CAD build for the part. Positions are in the model's coordinates, mm. Face numbers are marked on the shaded views. A direction names the side the tool comes from. Give positions to 0.01 mm unless a question says otherwise; leave off trailing zeros. Loops run counter-clockwise (first coordinate to the right, second up) from the corner with the lowest first, then second, coordinate; pieces in that order, holes last.
Item 1: Saw through at B-B on y = 1.5. Give the cut face in (x, z), plus the area to 3 significant figures.
Item 2: Probe probe 1 along X at (y, z) = (0.7, -29); probe 2 along X at (y, z) = (1.5, -29.5); probe 3 along Y at (x, z) = (37.5, -16.85). List the from-to ranges inside material, lowest first.
Item 3: Which spindle directions (+Z, -Z, +X, -X, +Y, -Y) get a long thin tool onto all of the face, cutting with end or side? Do the marked faces 1, 2 and 3. Say none if no direction does.
Item 4: Drop flat-ended pins along their axis: P1, Ø13, axis at y = 9, z = -20, coming from the +X side; P2, Ø4.5, axis at x = 20.5, y = 17, coming from the -Z side; P3, Ø2.5, axis at x = 49, z = -6, coming from the +Y side; P4, Ø5, axis at x = 17.5, y = 14.5, coming from the +Z side. Give the stop position or say it passes through.
Item 5: Saw through at D-D on x = 17.5. Give the cut face in (y, z), plus the area to 3 significant figures.
Item 6: Saw through at A-A on x = 6. Give the cut face in (y, z), plus the area to 3 significant figures.
Item 7: Saw through at C-C on z = -29. Give the cut face in (x, y).
from build123d import *

# Parameters (mm, degrees)
SKETCH_1_W          = 55
SKETCH_1_H          = 35
EXTRUDE_1_DEPTH     = 3
SKETCH_2_R          = 1.6
CUT_EXTRUDE_1_DEPTH = 3
FILLET_1_R          = 3
SKETCH_3_W          = 30
SKETCH_3_H          = 4
EXTRUDE_2_DEPTH     = 19
CHAMFER_1_SIZE      = 4
SKETCH_4_R          = 1.6
CUT_EXTRUDE_2_DEPTH = 19
FILLET_3_R          = 4


with BuildPart() as part:
    # 草图1 → 凸台-拉伸1 (new body)
    with BuildSketch(Plane(origin=(0, 0, 0), x_dir=(1, 0, 0), z_dir=(0, 1, 0))):
        with Locations((27.5, 17.5)):
            Rectangle(SKETCH_1_W, SKETCH_1_H)
    extrude(amount=EXTRUDE_1_DEPTH)

    # 草图2 → 切除-拉伸1 (cut)
    with BuildSketch(Plane(origin=(0, 3, 0), x_dir=(1, 0, 0), z_dir=(0, 1, 0))):
        with Locations(Location((6, 29, 0), (0, 0, 270))):
            Circle(SKETCH_2_R)
        with Locations(Location((49, 29, 0), (0, 0, 270))):
            Circle(SKETCH_2_R)
        with Locations(Location((49, 6, 0), (0, 0, 270))):
            Circle(SKETCH_2_R)
        with Locations(Location((6, 6, 0), (0, 0, 270))):
            Circle(SKETCH_2_R)
    extrude(amount=-CUT_EXTRUDE_1_DEPTH, mode=Mode.SUBTRACT)

    # 圆角1
    fillet_1_edges = [part.edges().sort_by_distance(p)[0] for p in [
        (0, 1.5, -35),
        (55, 1.5, -35),
        (55, 1.5, 0),
        (0, 1.5, 0),
    ]]
    fillet(fillet_1_edges, radius=FILLET_1_R)

    # 草图3 → 凸台-拉伸2 (add)
    with BuildSketch(Plane(origin=(0, 3, 0), x_dir=(1, 0, 0), z_dir=(0, 1, 0))):
        with Locations((27.5, 17.5)):
            Rectangle(SKETCH_3_W, SKETCH_3_H)
    extrude(amount=EXTRUDE_2_DEPTH)

    # 倒角1
    chamfer_1_edges = [part.edges().sort_by_distance(p)[0] for p in [
        (27.5, 3, -15.5),
        (27.5, 3, -19.5),
    ]]
    chamfer(chamfer_1_edges, length=CHAMFER_1_SIZE)

    # 草图4 → 切除-拉伸2 (cut)
    with BuildSketch(Plane(origin=(0, 0, -19.5), x_dir=(-1, 0, 0), z_dir=(0, 0, -1))):
        with Locations((-37.5, 14.5)):
            Circle(SKETCH_4_R)
        with Locations((-17.5, 14.5)):
            Circle(SKETCH_4_R)
    extrude(amount=-CUT_EXTRUDE_2_DEPTH, mode=Mode.SUBTRACT)

    # 圆角3
    fillet_3_edges = [part.edges().sort_by_distance(p)[0] for p in [
        (12.5, 22, -17.5),
        (42.5, 22, -17.5),
    ]]
    fillet(fillet_3_edges, radius=FILLET_3_R)


solid = part.part
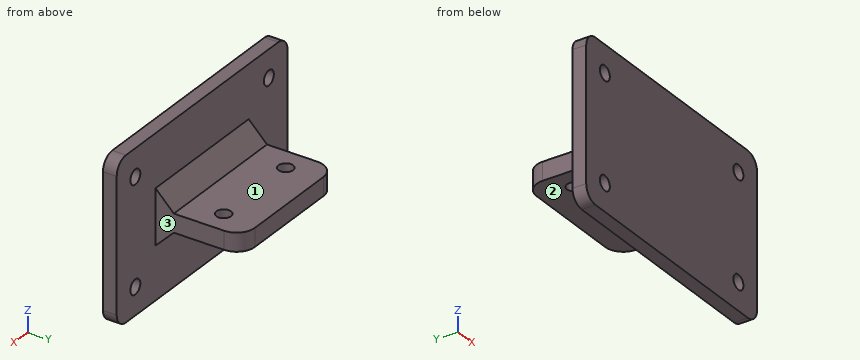
Results below:
1. outline: (0, -32) arc R3 ccw to (3, -35) - (52, -35) arc R3 ccw to (55, -32) - (55, -3) arc R3 ccw to (52, 0) - (3, 0) arc R3 ccw to (0, -3) - close; hole circle Ø3.2 at (6, -29); hole circle Ø3.2 at (6, -6); hole circle Ø3.2 at (49, -29); hole circle Ø3.2 at (49, -6)
1. area: 1,890 mm2
2. probe 1: x = 0 to 4.4, 7.6 to 47.4, 50.6 to 55
2. probe 2: x = 0 to 4.48, 7.52 to 47.48, 50.52 to 55
2. probe 3: y = 0 to 12.9, 16.1 to 22
3. face 1: +Z, +X, -X, +Y
3. face 2: -Z, +X, -X, +Y
3. face 3: +Z, -Z, +X, +Y
4. P1: stops at x = 55
4. P2: stops at z = -19.5
4. P3: passes through
4. P4: stops at z = -15.5
5. outline: (0, -35) - (3, -35) - (3, -23.5) - (7, -19.5) - (12.9, -19.5) - (12.9, -15.5) - (7, -15.5) - (3, -11.5) - (3, 0) - (0, 0) - close; (16.1, -19.5) - (22, -19.5) - (22, -15.5) - (16.1, -15.5) - close
5. area: 184 mm2
6. outline: (0, -35) - (3, -35) - (3, -30.6) - (0, -30.6) - close; (0, -27.4) - (3, -27.4) - (3, -7.6) - (0, -7.6) - close; (0, -4.4) - (3, -4.4) - (3, 0) - (0, 0) - close
6. area: 85.8 mm2
7. outline: (0, 0) - (4.4, 0) - (4.4, 3) - (0, 3) - close; (7.6, 0) - (47.4, 0) - (47.4, 3) - (7.6, 3) - close; (50.6, 0) - (55, 0) - (55, 3) - (50.6, 3) - close
